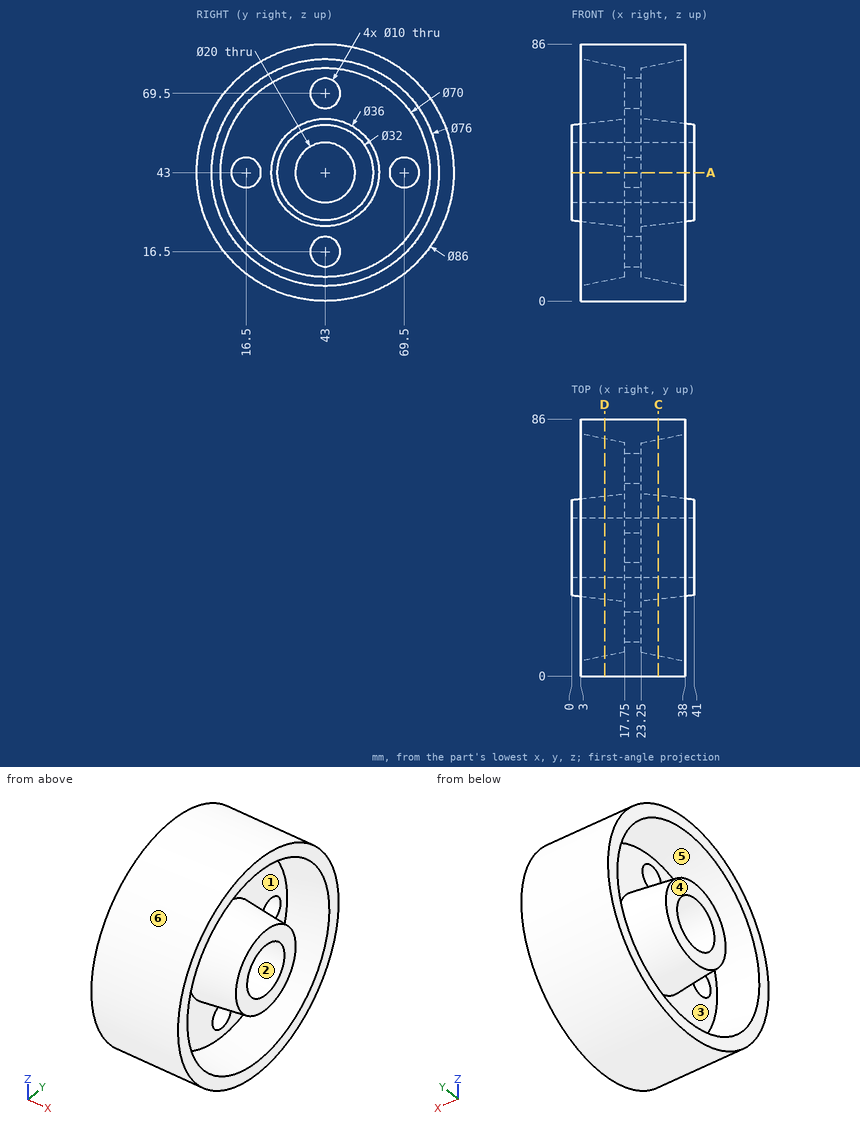
Source: three-view drawing plus pictorial views. Frame: mm from the lowest corner of the part. A direction names the side the tool comes from. Round coordinates to 2 decimals unless told otherwise and drop trailing zeros. Order: outer loops, then holes, each group sorted by start corner. A loop starts at its lowest first (then second) coordinate and runs counter-clockwise, first axis right, second up. Notation, with made-up numbers: (31.25, -9.5) -> (62.25, -9.5) arc R25 cw to (62.25, 26.5) -> close; hole circle Ø4 at (-16.75, 74.25). An arc over 180 degrees is marked (long way). Use CSV: the item, a comma, the result in double quotes. Start each with the question number.
1) Section A-A (z = 43). State how many separate pieces and enclosed holes the cut face has, and give its area (3 significant figures).
2) Draft query along Y for the marked faces 4, 5 and 6. Return one class per face: +Y half, -Y half, draft (parallel to the pull), parting line (faces both ways), or undercut.
3) Section D-D (x = 11). Return the cut outline in (y, z), and give its area (3 significant figures).
4) Material intervals for line 1 along Z through (x, y) = (20, 43); line 2 along Z through (x, y) = (14.5, 54.5), sorted ascending. Write a range as from..to.
5) Section C-C (x = 29). Return the cut outline in (y, z), and give its area (3 significant figures).
6) First-contact query: pin 1 Ø1 at (y, z) = (33.5, 73.5) entering from -X; pin 2 Ø8 at (y, z) = (38, 67) entering from +X; pin 3 Ø3 at (x, y) = (35, 67) entering from -Z. Flat tips, straight axial feed; report the tip coordinate or a pass-through.
7) Set-up query: the marked faces 1, 2 and 3. Return all of +Z, -Z, +X, -X, +Y, -Y with unobstructed straight access to the full face (end or side cutting, diameter ignored); none if empty.
Returned:
1,separate pieces,"4"
1,enclosed holes,"0"
1,area,"1,130 mm²"
2,face 4,"draft"
2,face 5,"undercut"
2,face 6,"parting line"
3,outline,"circle Ø86 at (43, 43); circle Ø34.48 at (43, 43); hole circle Ø72.75 at (43, 43); hole circle Ø20 at (43, 43)"
3,area,"2,270 mm²"
4,line 1,"z = 0..11.5, 21.5..33, 53..64.5, 74.5..86"
4,line 2,"z = 1.57..9.24, 29.63..56.37, 76.76..84.43"
5,outline,"circle Ø86 at (43, 43); circle Ø34.7 at (43, 43); hole circle Ø72.34 at (43, 43); hole circle Ø20 at (43, 43)"
5,area,"2,330 mm²"
6,pin 1,"stops at x = 17.75"
6,pin 2,"stops at x = 23.25"
6,pin 3,"stops at z = 6.36"
7,face 1,"+X"
7,face 2,"+X, -X"
7,face 3,"-X"
